```python
from build123d import *

# Parameters (mm, degrees)
F0_W     = 8
F0_H     = 4
F1_DEPTH = 4


with BuildPart() as f1:
    # F0 (on Right) → F1 (new body)
    with BuildSketch(Plane.YZ):
        with BuildLine():
            Line((0, 4), (0, 0))
            Line((0, 0), (50.8, 0))
            ThreePointArc((50.8, 0), (59.285281, 3.514719), (62.8, 12))
            ThreePointArc((62.8, 12), (61.628427, 14.828427), (58.8, 16))
            ThreePointArc((58.8, 16), (56.8, 14), (58.8, 12))
            ThreePointArc((58.8, 12), (56.456854, 6.343146), (50.8, 4))
            Line((50.8, 4), (47.8, 4))
            Line((47.8, 4), (37.8, 4))
            Line((37.8, 4), (13, 4))
            Line((13, 4), (3, 4))
            Line((3, 4), (0, 4))
        make_face()
        Polygon((3, 8), (3, 4), (13, 4), (13, 8), (12, 8), (4, 8), align=None)
        Polygon((37.8, 8), (37.8, 4), (47.8, 4), (47.8, 8), (46.8, 8), (38.8, 8), align=None)
        with Locations((8, 10)):
            Rectangle(F0_W, F0_H)
        with Locations((42.8, 10)):
            Rectangle(F0_W, F0_H)
    extrude(amount=F1_DEPTH)


solid = f1.part
```
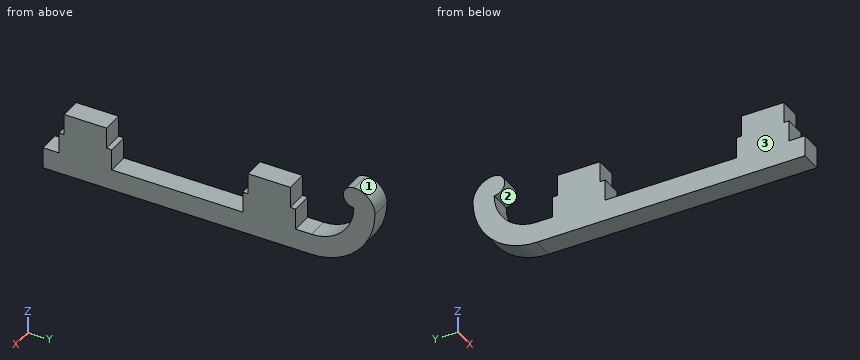
For this review, take the finished solid that the model builds, in its own axes (mm). Face numbers are marked on the shaded views. Round coordinates to 2 decimals unless told otherwise and drop trailing zeros. Write each loop counter-clockwise with the first axis right and the second up, starting at its lowest first coordinate (ties: lowest second). Pieces come first, ordered by that corner, then holes. Notation, with made-up numbers: (87.25, 76) -> (107.25, 76) arc R26 ccw to (107.25, 105) -> close; hole circle Ø6 at (5.25, 36.5). An arc over 180 degrees is marked (long way). One line per question, with ' | ' between items. Start each with the question number.
1) Add section B-B (y = 43). Write out the cut boundary in (x, z).
2) Add section A-A (x = 3.4). Write out the cut boundary in (y, z).
3) Add section C-C (z = 14.75). Write out the cut boundary in (x, y).
4) Mouldability with a two-part tool opening along Z and no side actions: class the marked faces 1, 2 and 3 as +Z half, -Z half, draft (parallel to the pull), parting line (faces both ways), or undercut.
5) Wall thickness on line 1 along Y through (x, z) = (0.2, 5); line 2 along Y through (x, z) = (3.25, 5.75); line 3 along Z through (x, y) = (3.4, 15): over which ranges is each line inside the solid? List them lowest first.
6) For pin 1 Ø1.1 at (x, y) = (2, 12.5) entering from +Z; pin 2 Ø2 at (x, z) = (1.5, 12.5) entering from -Y; pin 3 Ø1.2 at (x, z) = (2, 5.5) entering from +Y; pin 4 Ø8 at (y, z) = (52, 11.5) entering from -X, all flat-tipped, find the tip position at first contact; note any pin that passes through.
Reported:
1) outline: (0, 0) -> (4, 0) -> (4, 12) -> (0, 12) -> close
2) outline: (0, 0) -> (50.8, 0) arc R12 ccw to (62.8, 12) arc R4 ccw to (58.8, 16) arc R2 ccw to (58.8, 12) arc R8 cw to (50.8, 4) -> (47.8, 4) -> (47.8, 8) -> (46.8, 8) -> (46.8, 12) -> (38.8, 12) -> (38.8, 8) -> (37.8, 8) -> (37.8, 4) -> (13, 4) -> (13, 8) -> (12, 8) -> (12, 12) -> (4, 12) -> (4, 8) -> (3, 8) -> (3, 4) -> (0, 4) -> close
3) outline: (0, 56.95) -> (4, 56.95) -> (4, 61.7) -> (0, 61.7) -> close
4) face 1: +Z half | face 2: undercut | face 3: draft
5) line 1: y = 3 to 13, 37.8 to 47.8, 54.67 to 60.55 | line 2: y = 3 to 13, 37.8 to 47.8, 55.79 to 61.04 | line 3: z = 0 to 4
6) pin 1: stops at z = 12 | pin 2: stops at y = 4 | pin 3: stops at y = 61.25 | pin 4: passes through
